from build123d import *

# Parameters (mm, degrees)
SKETCH1_W               = 100
SKETCH1_H               = 100
BOSS_EXTRUDE1_DEPTH     = 5
SKETCH2_R               = 7.5
BOSS_EXTRUDE2_DEPTH     = 3
SKETCH3_R               = 2.5
BOSS_EXTRUDE3_DEPTH     = 3
CUT_EXTRUDE1_DEPTH      = 71.964779997
CUT_EXTRUDE2_DEPTH      = 12
CUT_EXTRUDE2_DEPTH_BACK = 5
SKETCH11_R              = 1
BOSS_EXTRUDE5_DEPTH     = 27
SHELL1_START            = 5.027136377
SHELL1_DEPTH            = 5
SHELL1_START_2          = -8.972863623
SHELL1_2_DEPTH          = 4
SHELL1_START_3          = 10.027136377
SHELL1_3_DEPTH          = 34.623982156
SHELL1_START_4          = 43.654391787
SHELL1_4_DEPTH          = 0.996726746
SHELL1_START_5          = 30.292722796
SHELL1_5_DEPTH          = 0.404221296
SHELL1_START_6          = 1
SHELL1_6_DEPTH          = 3
SHELL1_START_7          = -26
SHELL1_7_DEPTH          = 27
SHELL1_START_8          = 4
SHELL1_8_OUTLINE_R      = 6.5
SHELL1_8_DEPTH          = 3
SHELL1_START_9          = 7
SHELL1_9_OUTLINE_R      = 1.5
SHELL1_9_DEPTH          = 3
SHELL1_10_DEPTH         = 3
SKETCH14_W              = 105.332153784
SKETCH14_H              = 107.039050792
SKETCH14_R              = 50
CUT_EXTRUDE3_DEPTH      = 76.690157881
BOSS_EXTRUDE6_START     = -5
SKETCH15_R              = 50
SKETCH15_R_2            = 48.20184761
BOSS_EXTRUDE6_DEPTH     = 5
SKETCH16_W              = 2
SKETCH16_H              = 10
BOSS_EXTRUDE7_DEPTH     = 2


with BuildPart() as part:
    # Sketch1 → Boss-Extrude1 (new body)
    with BuildSketch(Plane.XY):
        Rectangle(SKETCH1_W, SKETCH1_H)
    extrude(amount=BOSS_EXTRUDE1_DEPTH)

    # Sketch2 → Boss-Extrude2 (add)
    with BuildSketch(Plane.XY.offset(5)):
        with Locations(Location((0, 0, 0), (0, 0, 180))):
            Circle(SKETCH2_R)
    extrude(amount=BOSS_EXTRUDE2_DEPTH)

    # Sketch3 → Boss-Extrude3 (add)
    with BuildSketch(Plane.XY.offset(8)):
        Circle(SKETCH3_R)
    extrude(amount=BOSS_EXTRUDE3_DEPTH)

    # Sketch10 → Cut-Extrude1 (cut, through all)
    with BuildSketch(Plane.XY.offset(5)):
        Polygon((-7.799279723, 15.528201009), (-13.921426992, 10.378510454), (-30.014209976, 29.510220671), (-23.892062707, 34.659911226), align=None)
    extrude(amount=-CUT_EXTRUDE1_DEPTH, mode=Mode.SUBTRACT)

    # Sketch11 → Cut-Extrude2 (cut, two sides: drawn at the far end of the back side and taken through both)
    with BuildSketch(Plane(origin=(3.081840247, 2.592313271, 0), x_dir=(0, 0, 1), z_dir=(-0.765268408666043, -0.6437113193798463, 0)).offset(-CUT_EXTRUDE2_DEPTH_BACK)):
        with Locations(Location((3.5, 20.903726316, 0), (0, 0, 90))):
            Circle(SKETCH11_R)
    extrude(amount=CUT_EXTRUDE2_DEPTH + CUT_EXTRUDE2_DEPTH_BACK, mode=Mode.SUBTRACT)

    # Sketch13 → Boss-Extrude5 (add)
    with BuildSketch(Plane(origin=(0, 0, 0), x_dir=(-1, 0, 0), z_dir=(0, 0, -1))):
        Polygon((-25.653340805, 17.18977508), (-37.06059478, 25.306089315), (-39.959278435, 21.232070039), (-28.552024461, 13.115755803), align=None)
    extrude(amount=BOSS_EXTRUDE5_DEPTH)

    # Shell1: read off the stored shape, not the designer's step
    # Shell1 outline → Shell1 (cut)
    with BuildSketch(Plane(origin=(0, 0, 0), x_dir=(0.6437113193798459, -0.7652684086660432, 0), z_dir=(0.7652684086660431, 0.6437113193798462, 0)).offset(SHELL1_START)):
        with BuildLine():
            Line((-18.967234643, -4), (-15.903726316, -4))
            Line((-15.903726316, -4), (-15.903726316, -1))
            Line((-15.903726316, -1), (-42.903726316, -1))
            Line((-42.903726316, -1), (-42.903726316, -4))
            Line((-42.903726316, -4), (-22.840217989, -4))
            ThreePointArc((-22.840217989, -4), (-20.903726316, -1.5), (-18.967234643, -4))
        make_face()
    extrude(amount=SHELL1_DEPTH, mode=Mode.SUBTRACT)

    # Shell1 2 outline → Shell1 2 (cut)
    with BuildSketch(Plane(origin=(0, 0, 0), x_dir=(0.6437113193798459, -0.7652684086660432, 0), z_dir=(0.7652684086660431, 0.6437113193798462, 0)).offset(SHELL1_START_2)):
        with BuildLine():
            Line((-18.967234643, -4), (-15.903726316, -4))
            Line((-15.903726316, -4), (-15.903726316, -1))
            Line((-15.903726316, -1), (-42.903726316, -1))
            Line((-42.903726316, -1), (-42.903726316, -4))
            Line((-42.903726316, -4), (-22.840217989, -4))
            ThreePointArc((-22.840217989, -4), (-20.903726316, -1.5), (-18.967234643, -4))
        make_face()
    extrude(amount=SHELL1_2_DEPTH, mode=Mode.SUBTRACT)

    # Shell1 3 outline → Shell1 3 (cut)
    with BuildSketch(Plane(origin=(0, 0, 0), x_dir=(0.6437113193798459, -0.7652684086660432, 0), z_dir=(0.7652684086660431, 0.6437113193798462, 0)).offset(SHELL1_START_3)):
        with BuildLine():
            Line((-22.840217989, -4), (-18.967234643, -4))
            ThreePointArc((-18.967234643, -4), (-20.903726316, -1.5), (-22.840217989, -4))
        make_face()
    extrude(amount=SHELL1_3_DEPTH, mode=Mode.SUBTRACT)

    # Shell1 4 outline → Shell1 4 (cut)
    with BuildSketch(Plane(origin=(0, 0, 0), x_dir=(0.6437113193798459, -0.7652684086660432, 0), z_dir=(0.7652684086660431, 0.6437113193798462, 0)).offset(SHELL1_START_4)):
        with BuildLine():
            Line((-18.967234643, -4), (-15.903726316, -4))
            Line((-15.903726316, -4), (-15.903726316, -1))
            Line((-15.903726316, -1), (-42.903726316, -1))
            Line((-42.903726316, -1), (-42.903726316, -4))
            Line((-42.903726316, -4), (-22.840217989, -4))
            ThreePointArc((-22.840217989, -4), (-20.903726316, -1.5), (-18.967234643, -4))
        make_face()
    extrude(amount=SHELL1_4_DEPTH, mode=Mode.SUBTRACT)

    # Shell1 5 outline → Shell1 5 (cut)
    with BuildSketch(Plane(origin=(0, 0, 0), x_dir=(0.6437113193798459, -0.7652684086660432, 0), z_dir=(0.7652684086660431, 0.6437113193798462, 0)).offset(SHELL1_START_5)):
        with BuildLine():
            Line((-18.967234643, -4), (-15.903726316, -4))
            Line((-15.903726316, -4), (-15.903726316, -1))
            Line((-15.903726316, -1), (-42.903726316, -1))
            Line((-42.903726316, -1), (-42.903726316, -4))
            Line((-42.903726316, -4), (-22.840217989, -4))
            ThreePointArc((-22.840217989, -4), (-20.903726316, -1.5), (-18.967234643, -4))
        make_face()
    extrude(amount=SHELL1_5_DEPTH, mode=Mode.SUBTRACT)

    # Shell1 6 outline → Shell1 6 (cut)
    with BuildSketch(Plane.XY.offset(SHELL1_START_6)):
        Polygon((49, -49), (49, 49), (17.13028231, 49), (23.932681775, 40.913049752), (23.169918284, 40.271445464), (15.827828511, 49), (-1.10407087, 49), (13.253992906, 31.930589712), (12.944655118, 31.670387888), (-1.632279393, 49), (-49, 49), (-49, -49), align=None)
        Polygon((-2.563957951, 18.625200517), (-6.390299995, 15.40664392), (-14.042984081, 8.969530726), (-17.104057716, 6.394685448), (-19.035191674, 8.690490674), (-21.610036952, 11.751564309), (-34.484263339, 27.056932482), (-31.423189704, 29.63177776), (-23.770505618, 36.068890954), (-19.944163574, 39.287447551), align=None, mode=Mode.SUBTRACT)
    extrude(amount=SHELL1_6_DEPTH, mode=Mode.SUBTRACT)

    # Shell1 7 outline → Shell1 7 (cut)
    with BuildSketch(Plane.XY.offset(SHELL1_START_7)):
        Polygon((36.245790924, 24.726352584), (26.46814466, 17.769511811), (29.366828316, 13.695492535), (39.14447458, 20.652333308), align=None)
    extrude(amount=SHELL1_7_DEPTH, mode=Mode.SUBTRACT)

    # Shell1 8 outline → Shell1 8 (cut)
    with BuildSketch(Plane.XY.offset(SHELL1_START_8)):
        Circle(SHELL1_8_OUTLINE_R)
    extrude(amount=SHELL1_8_DEPTH, mode=Mode.SUBTRACT)

    # Shell1 9 outline → Shell1 9 (cut)
    with BuildSketch(Plane.XY.offset(SHELL1_START_9)):
        Circle(SHELL1_9_OUTLINE_R)
    extrude(amount=SHELL1_9_DEPTH, mode=Mode.SUBTRACT)

    # Shell1 10 outline → Shell1 10 (add)
    with BuildSketch(Plane.XY.offset(SHELL1_START_6)):
        Polygon((15.827828511, 49), (17.13028231, 49), (16.289124734, 50), (14.986670935, 50), align=None)
        Polygon((-1.632279393, 49), (-1.10407087, 49), (-1.945228446, 50), (-2.473436969, 50), align=None)
    extrude(amount=SHELL1_10_DEPTH)

    # Sketch14 → Cut-Extrude3 (cut, through all)
    with BuildSketch(Plane(origin=(0, 0, 0), x_dir=(-1, 0, 0), z_dir=(0, 0, -1))):
        Rectangle(SKETCH14_W, SKETCH14_H)
        Circle(SKETCH14_R, mode=Mode.SUBTRACT)
    extrude(amount=-CUT_EXTRUDE3_DEPTH, mode=Mode.SUBTRACT)

    # Sketch15 → Boss-Extrude6 (add)
    with BuildSketch(Plane.XY.offset(5).offset(BOSS_EXTRUDE6_START)):
        with Locations(Location((0, 0, 0), (0, 0, 180))):
            Circle(SKETCH15_R)
        with Locations(Location((0, 0, 0), (0, 0, 180))):
            Circle(SKETCH15_R_2, mode=Mode.SUBTRACT)
    extrude(amount=BOSS_EXTRUDE6_DEPTH)

    # Sketch16 → Boss-Extrude7 (add)
    with BuildSketch(Plane(origin=(0, 0, 0), x_dir=(-1, 0, 0), z_dir=(0, 0, -1))):
        with Locations((25, 0)):
            Rectangle(SKETCH16_W, SKETCH16_H)
    extrude(amount=BOSS_EXTRUDE7_DEPTH)


solid = part.part
Work out the finished part from the listing and answer in its coordinate system (mm). A direction names the side the tool comes from. Give positions to 0.01 mm unless a question says otherwise; leave off trailing zeros. Loops run counter-clockwise (first coordinate to the right, second up) from the corner with the lowest first, then second, coordinate; pieces in that order, holes last. Notation, with made-up numbers: (48, 86) -> (56, 86) arc R36 cw to (56, 121) -> close; hole circle Ø7 at (79.5, 46). An arc over 180 degrees is marked (long way). Use a Markdown table: item, result. Add a question column.
1. Section A-A on z = -6 is taken. Determine the outline of the cut face in (x, y), and give its area (4 significant figures).
2. For faces 4 (the flat face through (27.123, 15.124, -13.311)), 5 (the flat face through (26.26, 17.62, -16.44)), 6 (the flat face through (-10.817, 12.989, 2.535)), 7 (the flat face through (-22.855, 19.445, 2.479)), 8 (the cylindrical face through (-0.54, -2.44, 9.48)), determine the directions among +Z, -Z, +X, -X, +Y, -Y from which every point of the face is accessible in a straight line to the end or side of a thin tool.
3. Determine the mould class of faces 1 (the flat face through (38.49, 23.3, -13.31)), 2 (the cylindrical face through (-47.69, 15.02, 2.46)), 3 (the flat face through (0, 0, 10)) for opening direction Y: released by +Y, released by -Y, zero draft, split by the parting line, or undercut.
4. Find the intervals of material crossed by probe 1 along Z at (x, y) = (-13, -17); probe 2 along Y at (x, z) = (0, 8.25); probe 3 along Y at (x, z) = (0, 7.85), in increasing order.
5. Flat-ended cylindrical pins translate along their axes: pin 1 Ø1.6 at (x, z) = (-25, -1.5) entering from -Y; pin 2 Ø0.6 at (x, z) = (-25, -0.5) entering from +Y; pin 3 Ø12 at (y, z) = (40, -10) entering from +X; pin 4 Ø5 at (x, y) = (-3.5, -38) entering from +Z. Find the tip coordinate at first contact, or state that the pin passes through.
6. Section D-D on y = -17.5 is taken. Determine the outline of the cut face in (x, z), and give its area (3 significant figures).
7. Section C-C on x = 23.5 is taken. Determine the outline of the cut face in (y, z), and give its area (3 significant figures).
8. Section B-B on y = 0 is taken. Determine the outline of the cut face in (x, z).
Results below:
| question | item | result |
|---|---|---|
| 1 | outline | (25.65, 17.19) -> (28.55, 13.12) -> (29.37, 13.7) -> (26.47, 17.77) -> close; (36.25, 24.73) -> (39.14, 20.65) -> (39.96, 21.23) -> (37.06, 25.31) -> close |
| 1 | area | 10.00 mm^2 |
| 2 | face 4 | -Z, -X, -Y |
| 2 | face 5 | -Z, -X, +Y |
| 2 | face 6 | +Z, -Z |
| 2 | face 7 | none |
| 2 | face 8 | +Z |
| 3 | face 1 | released by +Y |
| 3 | face 2 | split by the parting line |
| 3 | face 3 | undercut |
| 4 | probe 1 | z = 0 to 1, 4 to 5 |
| 4 | probe 2 | y = -2.5 to -1.5, 1.5 to 2.5 |
| 4 | probe 3 | y = -7.5 to -1.5, 1.5 to 7.5 |
| 5 | pin 1 | stops at y = -5 |
| 5 | pin 2 | stops at y = 5 |
| 5 | pin 3 | passes through |
| 5 | pin 4 | stops at z = 5 |
| 6 | outline | (-46.84, 0) -> (46.84, 0) -> (46.84, 5) -> (-46.84, 5) -> close; hole (-44.91, 1) -> (44.91, 1) -> (44.91, 4) -> (-44.91, 4) -> close |
| 6 | area | 199 mm^2 |
| 7 | outline | (-44.13, 0) -> (44.13, 0) -> (44.13, 5) -> (-44.13, 5) -> close; hole (-42.09, 1) -> (42.09, 1) -> (42.09, 4) -> (-42.09, 4) -> close |
| 7 | area | 189 mm^2 |
| 8 | outline | (-50, 0) -> (-26, 0) -> (-26, -2) -> (-24, -2) -> (-24, 0) -> (50, 0) -> (50, 5) -> (7.5, 5) -> (7.5, 8) -> (2.5, 8) -> (2.5, 11) -> (-2.5, 11) -> (-2.5, 8) -> (-7.5, 8) -> (-7.5, 5) -> (-50, 5) -> close; hole (-48.2, 1) -> (48.2, 1) -> (48.2, 4) -> (6.5, 4) -> (6.5, 7) -> (1.5, 7) -> (1.5, 10) -> (-1.5, 10) -> (-1.5, 7) -> (-6.5, 7) -> (-6.5, 4) -> (-48.2, 4) -> close |
